Geometry check sheet. Reference: drawing and pictorial views, mm from the part's lowest x, y, z. A direction names the side the tool comes from. Give positions to 0.01 mm unless a question says otherwise; leave off trailing zeros. Write each loop counter-clockwise with the first axis right and the second up, starting at its lowest first coordinate (ties: lowest second). Pieces come first, ordered by that corner, then holes. Notation, with made-up numbers: M 43.25,89.5 L 64.25,89.5 A8 ccw 64.25,100.5 Z; hole C -38.75,40.5 d8. An arc over 180 degrees is marked long. One line per item, written item: value. Start each with the question number.
1. Cross-section at B-B on y = 10.5. Record the cut outline in (x, z).
2. Tool access check on the marked faces 1 and 2. Record the directions out of +Z, -Z, +X, -X, +Y, -Y that give a thin tool (end or side, any length) a straight path to the whole face; none if there is none.
3. Gauge pin test, flat end, axial feed: pin 1 (2 mm diameter, centred on y = 14, z = 66, fed in from -X) (1 decimal). Record the tip position at first contact, or that the pin passes through.
4. Cross-section at C-C on z = 79. Record the cut outline in (x, y) (1 decimal).
5. Cross-section at A-A on x = 78.5. Record the cut outline in (y, z), then the cut area to 3 significant figures.
6. Scan lines: line 1 (Z direction, x = 24, y = 20.5); line 2 (Z direction, x = 29.5, y = 4.5) (1 decimal). Record each from-to range of solid material in increasing order.
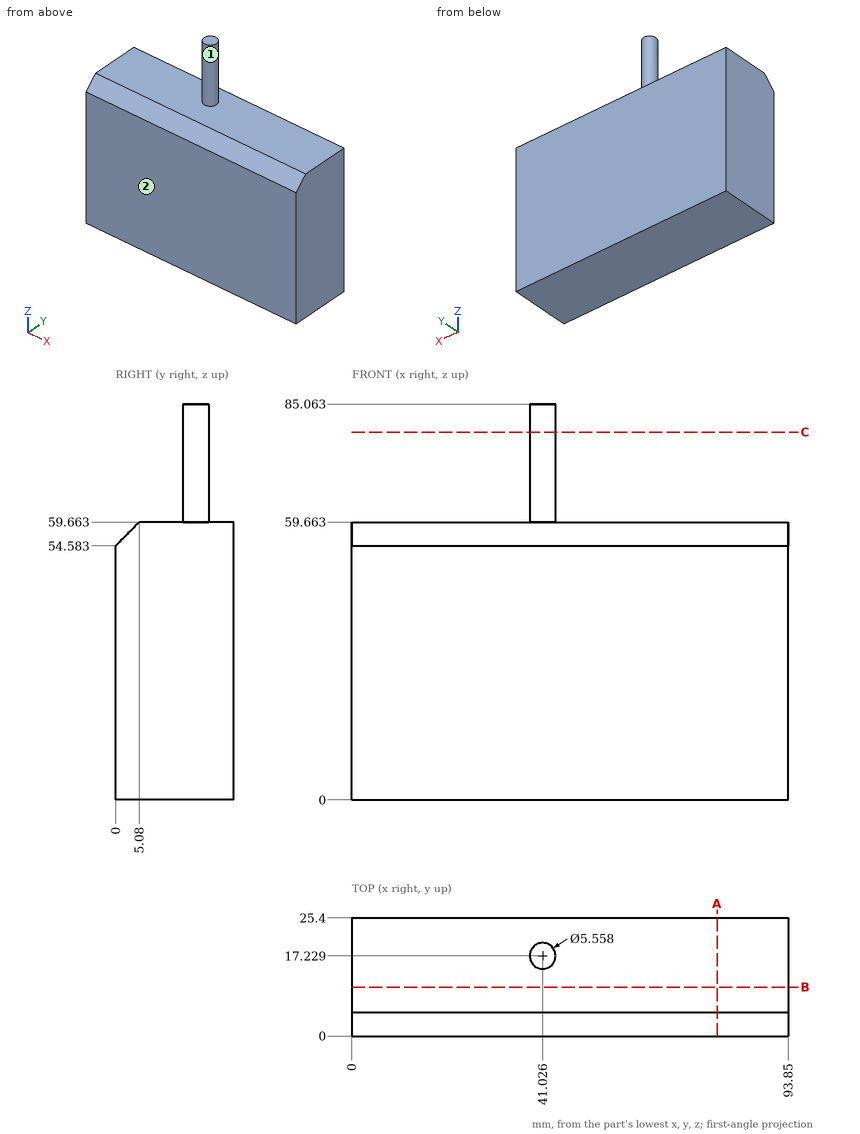
Report:
1. outline: M 0,0 L 93.85,0 L 93.85,59.66 L 0,59.66 Z
2. face 1: +Z
2. face 2: +Z, -Z, +X, -X, -Y
3. pin 1: stops at x = 39.4
4. outline: C 41,17.2 d5.6
5. outline: M 0,0 L 25.4,0 L 25.4,59.66 L 5.08,59.66 L 0,54.58 Z
5. area: 1,500 mm^2
6. line 1: z = 0 to 59.66
6. line 2: z = 0 to 59.1
